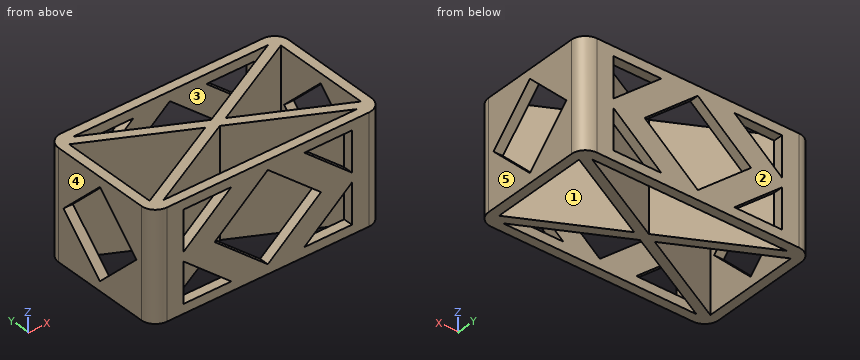
from build123d import *

# Parameters (mm, degrees)
F1_DEPTH = 23
F3_DEPTH = 40
F5_DEPTH = 60
F6_DEPTH = 23


with BuildPart() as f1:
    # F0 (on Top) → F1 (new body)
    with BuildSketch(Plane.XY):
        with BuildLine():
            ThreePointArc((-24.5, -10.75), (-23.62132, -12.87132), (-21.5, -13.75))
            Line((-21.5, -13.75), (21.5, -13.75))
            ThreePointArc((21.5, -13.75), (23.62132, -12.87132), (24.5, -10.75))
            Line((24.5, -10.75), (24.5, 10.75))
            ThreePointArc((24.5, 10.75), (23.62132, 12.87132), (21.5, 13.75))
            Line((21.5, 13.75), (-21.5, 13.75))
            ThreePointArc((-21.5, 13.75), (-23.62132, 12.87132), (-24.5, 10.75))
            Line((-24.5, 10.75), (-24.5, -10.75))
        make_face()
        with BuildLine():
            ThreePointArc((-21.5, -11.75), (-22.207107, -11.457107), (-22.5, -10.75))
            Line((-22.5, -10.75), (-22.5, -10.483528))
            Line((-22.5, -10.483528), (-22.5, 10.482972))
            Line((-22.5, 10.482972), (-22.5, 10.75))
            ThreePointArc((-22.5, 10.75), (-22.207107, 11.457107), (-21.5, 11.75))
            Line((-21.5, 11.75), (-20.593776, 11.75))
            Line((-20.593776, 11.75), (20.879046, 11.75))
            Line((20.879046, 11.75), (21.5, 11.75))
            ThreePointArc((21.5, 11.75), (22.207107, 11.457107), (22.5, 10.75))
            Line((22.5, 10.75), (22.5, 10.333408))
            Line((22.5, 10.333408), (22.5, -10.482972))
            Line((22.5, -10.482972), (22.5, -10.75))
            ThreePointArc((22.5, -10.75), (22.207107, -11.457107), (21.5, -11.75))
            Line((21.5, -11.75), (20.593776, -11.75))
            Line((20.593776, -11.75), (-20.586152, -11.75))
            Line((-20.586152, -11.75), (-21.5, -11.75))
        make_face(mode=Mode.SUBTRACT)
    extrude(amount=F1_DEPTH)

    # F2 (on face) → F3 (cut)
    with BuildSketch(Plane.XZ.offset(13.75)):
        Polygon((-17.908525, 12.5), (-7.778619, 21), (-17.908525, 21), align=None)
        Polygon((-11.321659, 11.5), (0, 2), (11.321659, 11.5), (0, 21), align=None)
        Polygon((-17.908525, 2), (-7.778619, 2), (-17.908525, 10.5), align=None)
        Polygon((17.908525, 10.5), (7.778619, 2), (17.908525, 2), align=None)
        Polygon((17.908525, 21), (7.778619, 21), (17.908525, 12.5), align=None)
    extrude(amount=-F3_DEPTH, mode=Mode.SUBTRACT)

    # F4 (on face) → F5 (cut)
    with BuildSketch(Plane.YZ.offset(24.5)):
        Polygon((-9.5, 11.5), (0, 2), (9.5, 11.5), (0, 21), align=None)
    extrude(amount=-F5_DEPTH, mode=Mode.SUBTRACT)

    # F0 (on Top) → F6 (join)
    with BuildSketch(Plane.XY):
        with BuildLine():
            Line((-22.5, -10.483528), (-22.5, -10.75))
            ThreePointArc((-22.5, -10.75), (-22.207107, -11.457107), (-21.5, -11.75))
            Line((-21.5, -11.75), (-20.586152, -11.75))
            Line((-20.586152, -11.75), (0.07148, -1.162122))
            Line((0.07148, -1.162122), (20.593776, -11.75))
            Line((20.593776, -11.75), (21.5, -11.75))
            ThreePointArc((21.5, -11.75), (22.207107, -11.457107), (22.5, -10.75))
            Line((22.5, -10.75), (22.5, -10.482972))
            Line((22.5, -10.482972), (2.259688, -0.040576))
            Line((2.259688, -0.040576), (22.5, 10.333408))
            Line((22.5, 10.333408), (22.5, 10.75))
            ThreePointArc((22.5, 10.75), (22.207107, 11.457107), (21.5, 11.75))
            Line((21.5, 11.75), (20.879046, 11.75))
            Line((20.879046, 11.75), (0.074486, 1.086815))
            Line((0.074486, 1.086815), (-20.593776, 11.75))
            Line((-20.593776, 11.75), (-21.5, 11.75))
            ThreePointArc((-21.5, 11.75), (-22.207107, 11.457107), (-22.5, 10.75))
            Line((-22.5, 10.75), (-22.5, 10.482972))
            Line((-22.5, 10.482972), (-2.113723, -0.034731))
            Line((-2.113723, -0.034731), (-22.5, -10.483528))
        make_face()
    extrude(amount=F6_DEPTH)


solid = f1.part
Geometry: final body of the model. Coordinates: model frame, mm. Face numbers are marked on the shaded views. A direction names the side the tool comes from. Give positions to 0.01 mm unless a question says otherwise; leave off trailing zeros. Write each loop counter-clockwise with the first axis right and the second up, starting at its lowest first coordinate (ties: lowest second). Pieces come first, ordered by that corner, then holes. Notation, with made-up numbers: (0, -30) -> (28, -30) arc R22 cw to (28, -23) -> close; hole circle Ø6 at (27.25, 9). An arc over 180 degrees is marked (long way). Answer in a Markdown table with one row per item.
(1) Section query C-C on y = 4.75. Return loops of the section in (x, z).
Answers below:
| item | result |
|---|---|
| outline | (-24.5, 0) -> (-22.5, 0) -> (-22.5, 6.75) -> (-24.5, 6.75) -> close; (-24.5, 16.25) -> (-22.5, 16.25) -> (-22.5, 23) -> (-24.5, 23) -> close; (-11.39, 0) -> (-7.03, 0) -> (-7.03, 23) -> (-11.39, 23) -> close; (7.22, 0) -> (11.61, 0) -> (11.61, 23) -> (7.22, 23) -> close; (22.5, 0) -> (24.5, 0) -> (24.5, 6.75) -> (22.5, 6.75) -> close; (22.5, 16.25) -> (24.5, 16.25) -> (24.5, 23) -> (22.5, 23) -> close |
(2) Draft query along X for the marked faces 3, 4 and 5. Return one class per face: +X half, -X half, draft (parallel to the pull), parting line (faces both ways), or undercut.
Answers below:
| item | result |
|---|---|
| face 3 | undercut |
| face 4 | -X half |
| face 5 | +X half |
(3) Section query B-B on x = 12. State how many separate pieces and enclosed holes the cut face has, then the cut area to 3 significant figures.
Answers below:
| item | result |
|---|---|
| separate pieces | 8 |
| enclosed holes | 0 |
| area | 167 mm^2 |
(4) Section query A-A on x = 19.5. Return loops of the section in (y, z), then the cut area to 3 significant figures.
Answers below:
| item | result |
|---|---|
| outline | (-13.75, 0) -> (-11.75, 0) -> (-11.75, 23) -> (-13.75, 23) -> close; (-11.19, 0) -> (-8.94, 0) -> (-8.94, 23) -> (-11.19, 23) -> close; (8.8, 0) -> (11.04, 0) -> (11.04, 23) -> (8.8, 23) -> close; (11.75, 0) -> (13.75, 0) -> (13.75, 23) -> (11.75, 23) -> close |
| area | 195 mm^2 |
(5) Section query D-D on x = -5. Return loops of the section in (y, z), then the cut area to 3 significant figures.
Answers below:
| item | result |
|---|---|
| outline | (-13.75, 0) -> (-11.75, 0) -> (-11.75, 6.2) -> (-13.75, 6.2) -> close; (-13.75, 16.8) -> (-11.75, 16.8) -> (-11.75, 23) -> (-13.75, 23) -> close; (-3.76, 0) -> (-1.51, 0) -> (-1.51, 23) -> (-3.76, 23) -> close; (1.45, 0) -> (3.7, 0) -> (3.7, 23) -> (1.45, 23) -> close; (11.75, 0) -> (13.75, 0) -> (13.75, 6.2) -> (11.75, 6.2) -> close; (11.75, 16.8) -> (13.75, 16.8) -> (13.75, 23) -> (11.75, 23) -> close |
| area | 153 mm^2 |
(6) Ray query, line 1 along X through (y, z) = (8.25, 3.5); line 2 along X through (y, z) = (8.75, 6.5); line 3 along Y through (x, z) = (14, 21.5). Return the intervals inside material, ascending. Write a range as [from, to].
Answers below:
| item | result |
|---|---|
| line 1 | [-24.5, -22.5], [-18.17, -13.81], [14.05, 18.44], [22.5, 24.5] |
| line 2 | [-24.5, -22.5], [-19.14, -14.78], [15.03, 19.41], [22.5, 24.5] |
| line 3 | [-13.75, -11.75], [-8.35, -6.1], [5.98, 8.22], [11.75, 13.75] |
(7) Pin query (flat end, axial travel): pin 1 (6.5 mm diameter, centred on y = 1, z = 15, fed in from +X); pin 2 (0.6 mm diameter, centred on y = 13, z = 16.5, fed in from +X); pin 3 (0.6 mm diameter, centred on y = 13, z = 17.5, fed in from -X); pin 4 (1 mm diameter, centred on x = 11, y = -9, fed in from +Z). Return the tip coordinate at first contact, or that it passes through.
Answers below:
| item | result |
|---|---|
| pin 1 | x = 10.63 |
| pin 2 | x = 23.78 |
| pin 3 | x = -23.78 |
| pin 4 | through |
(8) Set-up query: the marked faces 1 and 2. Return all of +Z, -Z, +X, -X, +Y, -Y with unobstructed straight access to the full face (end or side cutting, diameter ignored); none if empty.
Answers below:
| item | result |
|---|---|
| face 1 | +Z, -Z |
| face 2 | +Z, -Z, +X, -X, +Y |
